Geometry: final body of the model. Coordinates: model frame, mm. Face numbers are marked on the shaded views. A direction names the side the tool comes from. Round coordinates to 2 decimals unless told otherwise and drop trailing zeros. Loops run counter-clockwise (first coordinate to the right, second up) from the corner with the lowest first, then second, coordinate; pieces in that order, holes last. Notation, with made-up numbers: (67.25, 28) -> (81.25, 28) arc R15 ccw to (81.25, 54) -> close; hole circle Ø5 at (2.25, -22.5). An arc over 180 degrees is marked (long way). Answer in a Markdown table with one row per item.
```python
from build123d import *

# Parameters (mm, degrees)
BOSS_EXTRUDE2_DEPTH           = 12.7
FILLET1_R                     = 2
CSK_FOR_M5_SFHCS1_D           = 5.5
CSK_FOR_M5_SFHCS1_CSINK_D     = 11.2
CSK_FOR_M5_SFHCS1_CSINK_ANGLE = 90
M5_CLEARANCE_HOLE1_D          = 5.3
CUT_EXTRUDE1_DEPTH            = 4.5


with BuildPart() as part:
    # Sketch1 → Boss-Extrude2 (new body)
    with BuildSketch(Plane.XY):
        Polygon((0, -26.35), (0, -13.65), (5, -13.65), (5, 6.35), (37.6, 6.35), (37.6, -6.35), (15, -6.35), (15, -26.35), align=None)
    extrude(amount=BOSS_EXTRUDE2_DEPTH)

    # Fillet1
    fillet1_edges = [part.edges().sort_by_distance(p)[0] for p in [
        (5, -13.65, 6.35),
        (5, 6.35, 6.35),
        (37.6, 6.35, 6.35),
        (37.6, -6.35, 6.35),
        (15, -6.35, 6.35),
        (15, -26.35, 6.35),
    ]]
    fillet(fillet1_edges, radius=FILLET1_R)

    # CSK for M5 SFHCS1 (through all)
    with Locations(Plane(origin=(15, 0, 0), x_dir=(0, 0, -1), z_dir=(1, 0, 0))):
        with Locations((-6.35, -20)):
            CounterSinkHole(CSK_FOR_M5_SFHCS1_D / 2, CSK_FOR_M5_SFHCS1_CSINK_D / 2, counter_sink_angle=CSK_FOR_M5_SFHCS1_CSINK_ANGLE)

    # M5 Clearance Hole1 (through all)
    with Locations(Plane(origin=(37.6, 0, 0), x_dir=(0, 0, -1), z_dir=(1, 0, 0))):
        with Locations((-6.35, 0)):
            Hole(M5_CLEARANCE_HOLE1_D / 2)

    # Sketch8 → Cut-Extrude1 (cut)
    with BuildSketch(Plane(origin=(28.6, 0, 0), x_dir=(0, 0, -1), z_dir=(1, 0, 0))):
        Polygon((-12.7, 4.05), (-6.35, 4.05), (-4.01173141, 4.05), (-1.67346282, 0), (-4.01173141, -4.05), (-6.35, -4.05), (-12.7, -4.05), align=None)
    extrude(amount=CUT_EXTRUDE1_DEPTH, mode=Mode.SUBTRACT)


solid = part.part
```
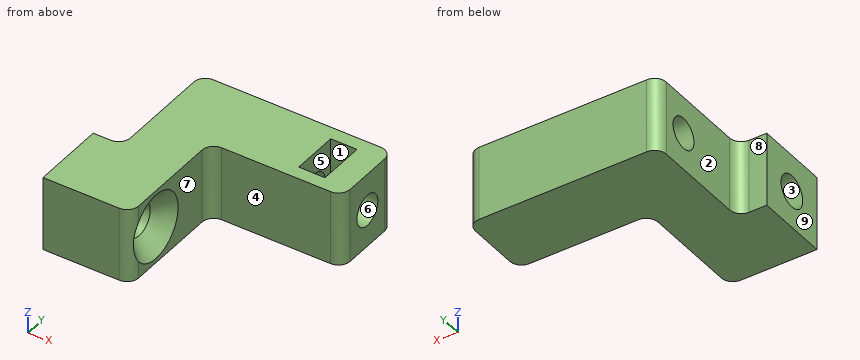
Item 1: Draft query along Y for the marked faces 1, 2, 3 and 4. Return one class per face: pulls with the +Y half, pulls with the -Y half, needs draft (parallel to the pull), parting line crosses it, or undercut.
Answer:
| item | result |
|---|---|
| face 1 | undercut |
| face 2 | needs draft |
| face 3 | undercut |
| face 4 | pulls with the -Y half |
Item 2: Line query: probe 1 along X at (y, z) = (3, 7.25); probe 2 along Y at (x, z) = (21.5, 6.35); probe 3 along Z at (x, y) = (7.25, -20). Output: solid intervals per line, ascending. Write a range as [from, to].
Answer:
| item | result |
|---|---|
| probe 1 | x = [5, 28.6], [33.1, 37.6] |
| probe 2 | y = [-6.35, -2.65], [2.65, 6.35] |
| probe 3 | z = [0, 3.6], [9.1, 12.7] |
Item 3: Cut plane C-C (x = 32). Output: boundary loops of the cut face in (y, z), then the cut area to 3 significant figures.
Answer:
| item | result |
|---|---|
| outline | (-6.35, 0) -> (6.35, 0) -> (6.35, 12.7) -> (4.05, 12.7) -> (4.05, 4.01) -> (0, 1.67) -> (-4.05, 4.01) -> (-4.05, 12.7) -> (-6.35, 12.7) -> close |
| area | 81.4 mm² |
Item 4: Reachability of the marked faces 5, 6, 7, 8 and 9 from +Z, -Z, +X, -X, +Y, -Y: full face, straight path, thin tool, end or side. Return the list, or none.
Answer:
| item | result |
|---|---|
| face 5 | +Z |
| face 6 | +X, -X |
| face 7 | +Z, -Z, +X, -Y |
| face 8 | +Z, -Z, -X, +Y |
| face 9 | +Z, -Z, -X, +Y, -Y |
Item 5: Cut plane A-A (y = -20). Output: boundary loops of the cut face in (x, z), then the cut area to 3 significant figures.
Answer:
| item | result |
|---|---|
| outline | (0, 0) -> (15, 0) -> (15, 0.75) -> (12.15, 3.6) -> (0, 3.6) -> close; (0, 9.1) -> (12.15, 9.1) -> (15, 11.95) -> (15, 12.7) -> (0, 12.7) -> close |
| area | 99.9 mm² |
Item 6: Cut plane D-D (x = 14.5). Output: boundary loops of the cut face in (y, z), then the cut area to 3 significant figures.
Answer:
| item | result |
|---|---|
| outline | (-25.67, 0) -> (6.35, 0) -> (6.35, 12.7) -> (-25.67, 12.7) -> close; hole circle Ø10.2 at (-20, 6.35); hole circle Ø5.3 at (0, 6.35) |
| area | 303 mm² |
Item 7: Cut plane B-B (z = 6.35). Count the separate pieces of the cut face and the enclosed holes in it, then the cut area to 3 significant figures.
Answer:
| item | result |
|---|---|
| separate pieces | 3 |
| enclosed holes | 0 |
| area | 400 mm² |
Item 8: Pin query (flat end, axial travel): pin 1 Ø5 at (x, z) = (30.5, 10.5) entering from -Y; pin 2 Ø2.5 at (y, z) = (0.5, 5) entering from -X; pin 3 Ø2.5 at (x, z) = (1, 9) entering from +Y. Return the tip coordinate at first contact, or that it passes through.
Answer:
| item | result |
|---|---|
| pin 1 | stops at y = -6.35 |
| pin 2 | stops at x = 5 |
| pin 3 | stops at y = -13.65 |
